Can you work these out from the model? Positions are in its coordinate system, mm. Coordinates: 2 decimals unless noted, no trailing zeros. Order: outer loops, then holes, each group sorted by start corner. A loop starts at its lowest first (then second) coordinate and runs counter-clockwise, first axis right, second up. Notation, with made-up numbers: (86, 6.5) -> (108, 6.5) arc R31 cw to (108, 34.5) -> close; hole circle Ø3 at (-40, 88.25). An arc over 180 degrees is marked (long way). Return JSON: item names as keys, results as strings. Group by question number.
1) If we section it at A-A, the plane y = -45.3: Please give me the cut outline in (x, z) (3 decimals), then the cut area to 3 significant figures.
2) If I drill on probe 1 along Y at (x, z) = (28.5, 2.35); probe 2 along Y at (x, z) = (56, 1); probe 3 along X at (y, z) = (28, 2.25), over which ranges is the centre line in solid material (lowest first)? Write a range as from..to.
3) If we section it at B-B, the plane y = 15.3: Please give me the cut outline in (x, z) (3 decimals), then the cut area to 3 significant figures.
4) If we section it at C-C, the plane y = -21.3: Please give me the cut outline in (x, z) (3 decimals), then the cut area to 3 significant figures.
5) For pin 1 (5 mm diameter, centred on x = -10.61, y = -31.41, fed in from -Z); pin 2 (1 mm diameter, centred on y = -33, z = 1.5, fed in from -X); pin 3 (1.5 mm diameter, centred on y = 17.5, z = 2, fed in from -X); pin 4 (0.9 mm diameter, centred on y = 32, z = 2, fed in from +X), each with a flat end and sliding along its axis, tell me the tip position at first contact or that it passes through.
6) If we section it at D-D, the plane z = 0.9: State how many separate pieces and enclosed holes the cut face has, then the cut area to 3 significant figures.
from build123d import *

# Parameters (mm, degrees)
ESQUISSE1_W             = 53.21
ESQUISSE1_H             = 101.6
ESQUISSE1_R             = 1.75
BOSS_EXTRU_1_DEPTH      = 3
ESQUISSE2_R             = 2.5
BOSS_EXTRU_2_DEPTH      = 3
ESQUISSE3_R             = 1.5
ENL_V_MAT_EXTRU_1_DEPTH = 3
ESQUISSE4_R             = 3
ENL_V_MAT_EXTRU_2_DEPTH = 4


with BuildPart() as part:
    # Esquisse1 → Boss.-Extru.1 (new body)
    with BuildSketch(Plane.XY):
        Rectangle(ESQUISSE1_W, ESQUISSE1_H)
        with Locations((-24.195, -35.5)):
            Circle(ESQUISSE1_R, mode=Mode.SUBTRACT)
        with Locations((24.065, -36.8)):
            Circle(ESQUISSE1_R, mode=Mode.SUBTRACT)
        with Locations((-8.995, 15.3)):
            Circle(ESQUISSE1_R, mode=Mode.SUBTRACT)
        with Locations((18.855, 15.3)):
            Circle(ESQUISSE1_R, mode=Mode.SUBTRACT)
        with Locations((-24.195, 39.43)):
            Circle(ESQUISSE1_R, mode=Mode.SUBTRACT)
        with Locations((24.065, 45.75)):
            Circle(ESQUISSE1_R, mode=Mode.SUBTRACT)
    extrude(amount=BOSS_EXTRU_1_DEPTH)

    # Esquisse2 → Boss.-Extru.2 (add)
    with BuildSketch(Plane.XY.offset(3)):
        with BuildLine():
            Line((0, 50.8), (0, 75.8))
            Line((0, 75.8), (-42.675883861, 75.8))
            ThreePointArc((-42.675883861, 75.8), (-49.604980355, 71.170125743), (-47.97918472, 62.996699141))
            ThreePointArc((-47.97918472, 62.996699141), (-47.97918472, 48.854563517), (-62.121320344, 48.854563517))
            ThreePointArc((-62.121320344, 48.854563517), (-70.294746945, 50.480359152), (-74.924621202, 43.551262658))
            Line((-74.924621202, 43.551262658), (-58.176555089, -42.706044052))
            ThreePointArc((-58.176555089, -42.706044052), (-54.721472053, -48.51558295), (-48.359885793, -50.8))
            Line((-48.359885793, -50.8), (-26.605, -50.8))
            Line((-26.605, -50.8), (-26.605, 50.8))
            Line((-26.605, 50.8), (0, 50.8))
        make_face()
        with Locations((-40.105, -45.3)):
            Circle(ESQUISSE2_R, mode=Mode.SUBTRACT)
        with Locations((-32.105, -21.3)):
            Circle(ESQUISSE2_R, mode=Mode.SUBTRACT)
        with Locations((-48.105, -21.3)):
            Circle(ESQUISSE2_R, mode=Mode.SUBTRACT)
        with Locations((-67.424621202, 43.551262658)):
            Circle(ESQUISSE2_R, mode=Mode.SUBTRACT)
        with Locations((-42.675883861, 68.3)):
            Circle(ESQUISSE2_R, mode=Mode.SUBTRACT)
        with BuildLine():
            Line((-61.174621202, 34.875473497), (-61.174621202, 26.875473497))
            ThreePointArc((-61.174621202, 26.875473497), (-62.924621202, 25.125473497), (-64.674621202, 26.875473497))
            Line((-64.674621202, 26.875473497), (-64.674621202, 34.875473497))
            ThreePointArc((-64.674621202, 34.875473497), (-62.924621202, 36.625473497), (-61.174621202, 34.875473497))
        make_face(mode=Mode.SUBTRACT)
        with BuildLine():
            Line((-61.174621202, 20.375473497), (-61.174621202, 12.375473497))
            ThreePointArc((-61.174621202, 12.375473497), (-62.924621202, 10.625473497), (-64.674621202, 12.375473497))
            Line((-64.674621202, 12.375473497), (-64.674621202, 20.375473497))
            ThreePointArc((-64.674621202, 20.375473497), (-62.924621202, 22.125473497), (-61.174621202, 20.375473497))
        make_face(mode=Mode.SUBTRACT)
        with BuildLine():
            Line((-34.0000947, 62.05), (-26.0000947, 62.05))
            ThreePointArc((-26.0000947, 62.05), (-24.2500947, 63.8), (-26.0000947, 65.55))
            Line((-26.0000947, 65.55), (-34.0000947, 65.55))
            ThreePointArc((-34.0000947, 65.55), (-35.7500947, 63.8), (-34.0000947, 62.05))
        make_face(mode=Mode.SUBTRACT)
        with BuildLine():
            Line((-19.5000947, 62.05), (-11.5000947, 62.05))
            ThreePointArc((-11.5000947, 62.05), (-9.7500947, 63.8), (-11.5000947, 65.55))
            Line((-11.5000947, 65.55), (-19.5000947, 65.55))
            ThreePointArc((-19.5000947, 65.55), (-21.2500947, 63.8), (-19.5000947, 62.05))
        make_face(mode=Mode.SUBTRACT)
    boss_extru_2 = extrude(amount=-BOSS_EXTRU_2_DEPTH)

    # Symétrie1: Boss.-Extru.2 across plane
    add(boss_extru_2.mirror(Plane(origin=(0, 50.8, 0), x_dir=(0, 0, 1), z_dir=(1, 0, 0))))

    # Esquisse3 → Enlèv. mat.-Extru.1 (cut)
    with BuildSketch(Plane.XY.offset(3)):
        with Locations((36.924621202, 34.875473497)):
            Circle(ESQUISSE3_R)
        with Locations((55.924621202, 34.875473497)):
            Circle(ESQUISSE3_R)
        with Locations((36.924621202, -2.124526503)):
            Circle(ESQUISSE3_R)
        with Locations((55.924621202, -2.124526503)):
            Circle(ESQUISSE3_R)
    extrude(amount=-ENL_V_MAT_EXTRU_1_DEPTH, mode=Mode.SUBTRACT)

    # Esquisse4 → Enlèv. mat.-Extru.2 (cut, through all)
    with BuildSketch(Plane.XY.offset(3)):
        with Locations((-10.606601718, -10.193398282)):
            Circle(ESQUISSE4_R)
        with Locations((10.606601718, -10.193398282)):
            Circle(ESQUISSE4_R)
        with Locations((-10.606601718, -31.406601718)):
            Circle(ESQUISSE4_R)
        with Locations((10.606601718, -31.406601718)):
            Circle(ESQUISSE4_R)
    extrude(amount=-ENL_V_MAT_EXTRU_2_DEPTH, mode=Mode.SUBTRACT)


solid = part.part
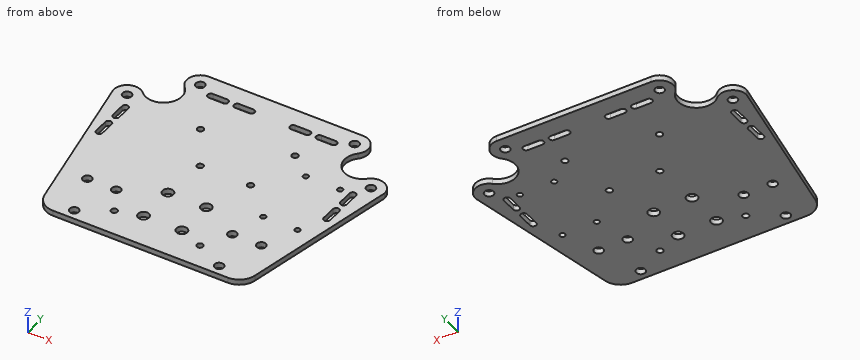
Result sheet:
{
 "1": {"outline": "(-57.29, 0) -> (-42.605, 0) -> (-42.605, 3) -> (-57.29, 3) -> close; (-37.605, 0) -> (37.605, 0) -> (37.605, 3) -> (-37.605, 3) -> close; (42.605, 0) -> (57.29, 0) -> (57.29, 3) -> (42.605, 3) -> close", "area": "314 mm2"},
 "2": {"probe 1": "y = -50.8..62.05, 65.55..75.8", "probe 2": "y = -47.25..-3.62, -0.63..33.38, 36.37..45.97", "probe 3": "x = -71.91..-64.67, -61.17..61.17, 64.67..71.91"},
 "3": {"outline": "(-69.439, 0) -> (-64.675, 0) -> (-64.675, 3) -> (-69.439, 3) -> close; (-61.175, 0) -> (-10.745, 0) -> (-10.745, 3) -> (-61.175, 3) -> close; (-7.245, 0) -> (17.105, 0) -> (17.105, 3) -> (-7.245, 3) -> close; (20.605, 0) -> (61.175, 0) -> (61.175, 3) -> (20.605, 3) -> close; (64.675, 0) -> (69.439, 0) -> (69.439, 3) -> (64.675, 3) -> close", "area": "375 mm2"},
 "4": {"outline": "(-62.333, 0) -> (-50.605, 0) -> (-50.605, 3) -> (-62.333, 3) -> close; (-45.605, 0) -> (-34.605, 0) -> (-34.605, 3) -> (-45.605, 3) -> close; (-29.605, 0) -> (29.605, 0) -> (29.605, 3) -> (-29.605, 3) -> close; (34.605, 0) -> (45.605, 0) -> (45.605, 3) -> (34.605, 3) -> close; (50.605, 0) -> (62.333, 0) -> (62.333, 3) -> (50.605, 3) -> close", "area": "314 mm2"},
 "5": {"pin 1": "passes through", "pin 2": "stops at x = -60.16", "pin 3": "stops at x = -70.01", "pin 4": "stops at x = 72.77"},
 "6": {"separate pieces": "1", "enclosed holes": "32", "area": "15,000 mm2"}
}
